from build123d import *

# Parameters (mm, degrees)
SKETCH1_R                   = 1.5
BOSS_EXTRUDE1_DEPTH         = 1.6
FILLET1_R                   = 3
FILLET2_R                   = 3
SKETCH2_R                   = 2.75
SCREW_HEADS_DEPTH           = 2
SCREW_HEADS_DRAFT           = -45
SCREW_HEADS_PROFILE_2_DEPTH = 2
SCREW_HEADS_PROFILE_2_DRAFT = -45
SKETCH3_W                   = 1
SKETCH3_H                   = 15
AIR_VENTS_DEPTH             = 2


with BuildPart() as part:
    # Sketch1 → Boss-Extrude1 (new body)
    with BuildSketch(Plane.XY):
        Polygon((-42.5, 43.777330307), (42.5, 43.777330307), (42.5, 40.777330307), (46.5, 38.467511309), (46.5, 32.177265409), (42.5, 28.777330307), (38.5, 28.777330307), (36.5, 26.777330307), (36.5, 17.277330307), (-36.5, 17.277330307), (-36.5, 26.777330307), (-38.5, 28.777330307), (-42.5, 28.777330307), (-46.5, 32.177265409), (-46.5, 38.467511309), (-42.5, 40.777330307), align=None)
        with Locations((-43, 35.322388359)):
            Circle(SKETCH1_R, mode=Mode.SUBTRACT)
        with Locations(Location((43, 35.322388359, 0), (0, 0, 180))):
            Circle(SKETCH1_R, mode=Mode.SUBTRACT)
    extrude(amount=BOSS_EXTRUDE1_DEPTH)

    # Fillet1
    fillet1_edges = [part.edges().sort_by_distance(p)[0] for p in [
        (42.5, 43.777330307, 0.8),
    ]]
    fillet(fillet1_edges, radius=FILLET1_R - 0.0001)  # a hair under: the kernel refuses the full size

    # Fillet2
    fillet2_edges = [part.edges().sort_by_distance(p)[0] for p in [
        (-42.5, 43.777330307, 0.8),
    ]]
    fillet(fillet2_edges, radius=FILLET2_R - 0.0001)  # a hair under: the kernel refuses the full size


with BuildPart() as screw_heads_tool:
    # Sketch2 → Screw Heads (with draft: the straight prism first)
    with BuildSketch(Plane.XY.offset(1.6)):
        with Locations((-43, 35.322388359)):
            Circle(SKETCH2_R)
    extrude(amount=-SCREW_HEADS_DEPTH)
    # Screw Heads: the draft: its side faces are tilted about the plane it starts from
    screw_heads_sides = [screw_heads_tool.faces().sort_by_distance(p)[0] for p in [
        (-45.75, 35.322388359, 0.6),
    ]]
    draft(screw_heads_sides, Plane.XY.offset(1.6), SCREW_HEADS_DRAFT)


with BuildPart() as part_1:
    add(part.part)

    # Screw Heads: cut by screw_heads_tool
    add(screw_heads_tool.part, mode=Mode.SUBTRACT)


with BuildPart() as screw_heads_profile_2_tool:
    # Sketch2 → Screw Heads profile 2 (with draft: the straight prism first)
    with BuildSketch(Plane.XY.offset(1.6)):
        with Locations((43, 35.322388359)):
            Circle(SKETCH2_R)
    extrude(amount=-SCREW_HEADS_PROFILE_2_DEPTH)
    # Screw Heads profile 2: the draft: its side faces are tilted about the plane it starts from
    screw_heads_profile_2_sides = [screw_heads_profile_2_tool.faces().sort_by_distance(p)[0] for p in [
        (40.25, 35.322388359, 0.6),
    ]]
    draft(screw_heads_profile_2_sides, Plane.XY.offset(1.6), SCREW_HEADS_PROFILE_2_DRAFT)


with BuildPart() as part_2:
    add(part_1.part)

    # Screw Heads profile 2: cut by screw_heads_profile_2_tool
    add(screw_heads_profile_2_tool.part, mode=Mode.SUBTRACT)

    # Sketch3 → Air Vents (cut)
    with BuildSketch(Plane.XY.offset(1.6)):
        with Locations((-26, 31.277330307)):
            Rectangle(SKETCH3_W, SKETCH3_H)
        with Locations((-20, 31.277330307)):
            Rectangle(SKETCH3_W, SKETCH3_H)
        with Locations((-14, 31.277330307)):
            Rectangle(SKETCH3_W, SKETCH3_H)
        with Locations((-8, 31.277330307)):
            Rectangle(SKETCH3_W, SKETCH3_H)
        with Locations((8, 31.277330307)):
            Rectangle(SKETCH3_W, SKETCH3_H)
        with Locations((14, 31.277330307)):
            Rectangle(SKETCH3_W, SKETCH3_H)
        with Locations((20, 31.277330307)):
            Rectangle(SKETCH3_W, SKETCH3_H)
        with Locations((26, 31.277330307)):
            Rectangle(SKETCH3_W, SKETCH3_H)
    extrude(amount=-AIR_VENTS_DEPTH, mode=Mode.SUBTRACT)


solid = part_2.part
Design review of the part built by this model. Coordinates are the model's own, in mm. A direction names the side the tool comes from. Coordinates: 2 decimals unless noted, no trailing zeros. One line per item, written item: value.
1) Add section A-A (z = 1.2). Give the number of separate pieces and of enclosed holes in the cut face, plus the area to 3 significant figures.
Answer sheet:
separate pieces: 1
enclosed holes: 10
area: 2,030 mm2
2) To check wall thickness, follow probe 1 along X at (y, z) = (22.75, 0.8); probe 2 along Y at (x, z) = (43, 0.15); probe 3 along Y at (x, z) = (39, 1.35). State the ranges of each line that lie inside material, in increasing order.
Answer sheet:
probe 1: x = -36.5 to 36.5
probe 2: y = 29.2 to 33.82, 36.82 to 40.49
probe 3: y = 28.78 to 43.78
3) For faces 4 (the face through (-44.47, 30.45, 0.79)), 5 (the face through (-8.5, 31, 1)), list the 3-axis set-ups (+Z, -Z, +X, -X, +Y, -Y) from which the entire face can be reached by the end or side of a thin tool; tool diameter is ignored.
Answer sheet:
face 4: +Z, -Z, -X, -Y
face 5: +Z, -Z
4) Mouldability with a two-part tool opening along Y and no side actions: class faces 1 (the face through (-41.6, 42.92, 0.81)), 2 (the face through (-13.5, 31, 1)), 3 (the face through (37.51, 27.79, 0.79)) as +Y half, -Y half, draft (parallel to the pull), parting line (faces both ways), or undercut.
Answer sheet:
face 1: +Y half
face 2: undercut
face 3: -Y half
5) Insertion check: pin 1 (3 mm diameter, centred on x = -24.5, y = 36, fed in from -Z); pin 2 (0.5 mm diameter, centred on y = 29, z = 0.5, fed in from -X); pin 3 (0.8 mm diameter, centred on y = 29, z = 1, fed in from +X); pin 4 (0.8 mm diameter, centred on y = 28.5, z = 1, fed in from -X). Each pin has a flat end and moves straight along its axis. Give the tip position at first contact, or say it passes through.
Answer sheet:
pin 1: stops at z = 0
pin 2: stops at x = -43.06
pin 3: stops at x = 43.23
pin 4: stops at x = -42.64
